```python
from build123d import *

# Parameters (mm, degrees)
SKETCH1_W                = 16.760563381
SKETCH1_H                = 70
BOSS_EXTRUDE1_DEPTH      = 10
SKETCH1_3_R              = 3
CUT_EXTRUDE1_DEPTH       = 20
BOSS_EXTRUDE2_DEPTH      = 10
SKETCH9_R                = 24.999512183
CUT_EXTRUDE4_DEPTH       = 11
BOSS_EXTRUDE4_DEPTH      = 5
BOSS_EXTRUDE4_DEPTH_BACK = 10


with BuildPart() as part:
    # Sketch1 → Boss-Extrude1 (new body)
    with BuildSketch(Plane(origin=(0, 0, 0), x_dir=(1, 0, 0), z_dir=(0, 1, 0))):
        with Locations((-61.126760563, 24.401408451)):
            Rectangle(SKETCH1_W, SKETCH1_H)
    extrude(amount=-BOSS_EXTRUDE1_DEPTH)

    # Sketch1_3 → Cut-Extrude1 (cut)
    with BuildSketch(Plane(origin=(0, 0, 0), x_dir=(1, 0, 0), z_dir=(0, 1, 0))):
        with Locations(Location((-61.126760563, 49.401408451, 0), (0, 0, 270))):
            Circle(SKETCH1_3_R)
        with Locations(Location((-61.126760563, -0.598591549, 0), (0, 0, 270))):
            Circle(SKETCH1_3_R)
    extrude(amount=-CUT_EXTRUDE1_DEPTH, mode=Mode.SUBTRACT)


with BuildPart() as body_2:
    # Sketch3 → Boss-Extrude2 (new body)
    with BuildSketch(Plane(origin=(-10.44184171, 0, 0), x_dir=(1, 0, 0), z_dir=(0, 1, 0))):
        with BuildLine():
            Line((-0.685894488, 46.401408451), (-0.685894488, 24.401408451))
            Line((-0.685894488, 24.401408451), (7.694387203, 24.401408451))
            Line((7.694387203, 24.401408451), (7.694387203, 59.401408451))
            Line((7.694387203, 59.401408451), (-0.685894488, 59.401408451))
            Line((-0.685894488, 59.401408451), (-0.685894488, 52.401408451))
            ThreePointArc((-0.685894488, 52.401408451), (1.435425856, 51.522728794), (2.314105512, 49.401408451))
            ThreePointArc((2.314105512, 49.401408451), (1.435425856, 47.280088107), (-0.685894488, 46.401408451))
        make_face()
        with BuildLine():
            Line((-9.066176178, 24.401408451), (-0.685894488, 24.401408451))
            Line((-0.685894488, 24.401408451), (-0.685894488, 46.401408451))
            ThreePointArc((-0.685894488, 46.401408451), (-3.685894488, 49.401408451), (-0.685894488, 52.401408451))
            Line((-0.685894488, 52.401408451), (-0.685894488, 59.401408451))
            Line((-0.685894488, 59.401408451), (-9.066176178, 59.401408451))
            Line((-9.066176178, 59.401408451), (-9.066176178, 24.401408451))
        make_face()
        with BuildLine():
            Line((-0.685894488, 2.401408451), (-0.685894488, 24.401408451))
            Line((-0.685894488, 24.401408451), (-9.066176178, 24.401408451))
            Line((-9.066176178, 24.401408451), (-9.066176178, -10.598591549))
            Line((-9.066176178, -10.598591549), (-0.685894488, -10.598591549))
            Line((-0.685894488, -10.598591549), (-0.685894488, -3.598591549))
            ThreePointArc((-0.685894488, -3.598591549), (-3.685894488, -0.598591549), (-0.685894488, 2.401408451))
        make_face()
        with BuildLine():
            Line((7.694387203, 24.401408451), (-0.685894488, 24.401408451))
            Line((-0.685894488, 24.401408451), (-0.685894488, 2.401408451))
            ThreePointArc((-0.685894488, 2.401408451), (1.435425856, 1.522728794), (2.314105512, -0.598591549))
            ThreePointArc((2.314105512, -0.598591549), (1.435425856, -2.719911893), (-0.685894488, -3.598591549))
            Line((-0.685894488, -3.598591549), (-0.685894488, -10.598591549))
            Line((-0.685894488, -10.598591549), (7.694387203, -10.598591549))
            Line((7.694387203, -10.598591549), (7.694387203, 24.401408451))
        make_face()
    extrude(amount=-BOSS_EXTRUDE2_DEPTH)


with BuildPart() as cut_extrude4_tool:
    # Sketch9 → Cut-Extrude4 (new body)
    with BuildSketch(Plane(origin=(0, 0, 0), x_dir=(1, 0, 0), z_dir=(0, 1, 0))):
        with Locations((-36.12724838, 24.401408451)):
            Circle(SKETCH9_R)
    extrude(amount=-CUT_EXTRUDE4_DEPTH)


with BuildPart() as part_1:
    add(part.part)

    # Cut-Extrude4: cut by cut_extrude4_tool
    add(cut_extrude4_tool.part, mode=Mode.SUBTRACT)



with BuildPart() as body_2_1:
    add(body_2.part)

    # Cut-Extrude4: cut by cut_extrude4_tool
    add(cut_extrude4_tool.part, mode=Mode.SUBTRACT)


with BuildPart() as part_2:
    add(part_1.part)

    add(body_2_1.part)  # Boss-Extrude4 merges body 2
    # Sketch8 → Boss-Extrude4 (add, two sides: drawn at the far end of the back side and taken through both)
    with BuildSketch(Plane(origin=(0, 0, 0), x_dir=(1, 0, 0), z_dir=(0, 1, 0)).offset(-BOSS_EXTRUDE4_DEPTH_BACK)):
        with BuildLine():
            Line((-2.747454507, 59.401408451), (-2.747454507, -10.598591549))
            Line((-2.747454507, -10.598591549), (-19.508017888, -10.598591549))
            Line((-19.508017888, -10.598591549), (-52.746478873, -10.598591549))
            Line((-52.746478873, -10.598591549), (-69.507042254, -10.598591549))
            Line((-69.507042254, -10.598591549), (-69.507042254, 59.401408451))
            ThreePointArc((-69.507042254, 59.401408451), (-139.507042254, -10.598591549), (-69.507042254, -80.598591549))
            Line((-69.507042254, -80.598591549), (-2.747454507, -80.598591549))
            ThreePointArc((-2.747454507, -80.598591549), (67.252545493, -10.598591549), (-2.747454507, 59.401408451))
        make_face()
    extrude(amount=BOSS_EXTRUDE4_DEPTH + BOSS_EXTRUDE4_DEPTH_BACK)


solid = part_2.part
```
Work out the finished part from the listing and answer in its coordinate system (mm). A direction names the side the tool comes from. Round coordinates to 2 decimals unless told otherwise and drop trailing zeros. Loops run counter-clockwise (first coordinate to the right, second up) from the corner with the lowest first, then second, coordinate; pieces in that order, holes last.
(1) The part is cut by section A-A, the plane y = -4.25. Give the vertices of the cut face in (x, z), and give its area (3 significant figures).
Computed values:
outline: (-69.51, -59.4) - (-52.75, -59.4) - (-52.75, -43.08) arc R25 cw to (-52.75, -5.73) - (-52.75, 10.6) - (-19.51, 10.6) - (-19.51, -5.73) arc R25 cw to (-19.51, -43.08) - (-19.51, -59.4) - (-2.75, -59.4) arc R70 ccw to (-2.75, 80.6) - (-69.51, 80.6) arc R70 ccw to start; hole circle Ø6 at (-61.13, -49.4); hole circle Ø6 at (-61.13, 0.6); hole circle Ø6 at (-11.13, -49.4); hole circle Ø6 at (-11.13, 0.6)
area: 21,900 mm2
(2) Find the intervals of material crossed by L1, parallel to X at y = -8.75, z = 9; L2, parallel to Z at x = -44.5, y = -3; L3, parallel to X at y = -5.25, z = -10, in increasing order.
Computed values:
L1: x = -139.49 to -52.75, -19.51 to 67.23
L2: z = 10.6 to 80.6
L3: x = -136.41 to -56.56, -15.69 to 64.15
(3) The part is cut by section C-C, the plane x = -113. Give the vertices of the cut face in (y, z).
Computed values:
outline: (-10, -44.25) - (5, -44.25) - (5, 65.45) - (-10, 65.45) - close
(4) The part is cut by section B-B, the plane z = -39. Give the vertices of the cut face in (x, y), and give its area (3 significant figures).
Computed values:
outline: (-118.9, -10) - (-56.42, -10) - (-56.42, 0) - (-69.51, 0) - (-69.51, 5) - (-118.9, 5) - close; (-15.83, -10) - (46.65, -10) - (46.65, 5) - (-2.75, 5) - (-2.75, 0) - (-15.83, 0) - close
area: 1,740 mm2
(5) For faces 1 (the flat face through (-61, -5, -59.401)), 2 (the flat face through (-52.746, -5, 3)), 3 (the flat face through (-2.747, 2, -25)), determine the directions among +Z, -Z, +X, -X, +Y, -Y from which every point of the face is accessible in a straight line to the end or side of a thin tool.
Computed values:
face 1: -Z, +X, -X, +Y, -Y
face 2: -Z, +Y, -Y
face 3: -Z, +Y
(6) The mould has two halves that part along Z. Classify faces 4 (the cylindrical face through (-11.13, -4.93, -24.11)), 5 (the flat face through (-11, -5, -59.401)), 6 (the flat face through (-19.508, -5, -51)), 7 (the cylindrical face through (-58.152, -4.93, 0.208)): pulls with the +Z half, pulls with the -Z half, needs draft (parallel to the pull), parting line crosses it, or undercut.
Computed values:
face 4: undercut
face 5: pulls with the -Z half
face 6: needs draft
face 7: undercut
(7) The part is cut by section D-D, the plane z = 39.5. Give the vertices of the cut face in (x, y).
Computed values:
outline: (-133.26, -10) - (61.01, -10) - (61.01, 5) - (-133.26, 5) - close
(8) Each of these flat-tipped pins is pushed along its axis until it touches: P1, Ø1.5, axis at y = -6.5, z = -19, coming from the +X side; P2, Ø8, axis at y = -3, z = -52.5, coming from the +X side; P3, Ø8, axis at x = -74.5, y = 2.5, coming from the +Z side; P4, Ø5.5, axis at x = -61.13, z = 0.6, coming from the -Y side. Where does it stop, or does it pass through?
Computed values:
P1: stops at x = 61.03
P2: stops at x = 34.77
P3: stops at z = 80.59
P4: passes through
